Autodesk Inventor part; units mm, degrees
ref_plane "YZ Plane" through (0, 0, 0) normal (1, 0, 0) x (0, 1, 0)
ref_plane "XZ Plane" through (0, 0, 0) normal (0, 1, 0) x (-1, 0, 0)
ref_plane "XY Plane" through (0, 0, 0) normal (0, 0, 1) x (1, 0, 0)
sketch "Boceto2" plane through (0, 0, 0) normal (0, 0, 1) x (1, 0, 0)
  line L0 (-14, 15) -> (0, 15)
  line L1 (3, 8.5) -> (3, 3.5)
  line L2 (0, 0) -> (-14, 0)
  line L3 (-17, 3.5) -> (-17, 8.5)
  line L4 (-14, 8.5) -> (-17, 8.5)
  line L5 (-17, 3.5) -> (-14, 3.5)
  line L6 (0, 8.5) -> (3, 8.5)
  line L7 (0, 3.5) -> (3, 3.5)
  line L8 (-14, 15) -> (-14, 8.5)
  line L9 (-14, 3.5) -> (-14, 0)
  line L10 (0, 15) -> (0, 8.5)
  line L11 (0, 3.5) -> (0, 0)
  point P0 (1.5, 3.5)
  dimension "d4" = 20
  dimension "d5" = 15
  dimension "d9" = 5
  dimension "d10" = 3
  dimension "d11" = 3
  dimension "d12" = 5
  dimension "d15" = 3.5
extrude "Extrusión1" add sketch "Boceto2" along normal blind 3
properties part number "abajo"
Source: CAD feature listing. Evaluate the final solid. Frame: model axes, mm. A direction names the side the tool comes from. Give positions to 0.01 mm unless a question says otherwise; leave off trailing zeros. Order: outer loops, then holes, each group sorted by start corner. A loop starts at its lowest first (then second) coordinate and runs counter-clockwise, first axis right, second up.
(1) Material intervals for line 1 along Y through (x, z) = (-14.75, 0.2); line 2 along X through (y, z) = (1.75, 1.2), sorted ascending.
(2) Section query A-A (z = 1.6). Return the cut outline in (x, y).
(3) Access query for faces 4 (the face through (-15, 8.5, 1)), 5 (the face through (-16, 3.5, 1)), 6 (the face through (0, 12, 1)), 7 (the face through (1, 3.5, 1)), 8 (the face through (-7, 0, 1)). Directions: +Z, -Z, +X, -X, +Y, -Y. A direction counts if a zero-diameter tool reaches every point of the face in a straight line with its end or side. Return the directions, or none.
(4) Contact query for flat-ended pins moving along their axis: P1, Ø1.5, axis at y = 11.5, z = 1, coming from the +X side; P2, Ø1.5, axis at y = 1, z = 1.5, coming from the -X side; P3, Ø1.5, axis at x = 2, z = 1, coming from the +Y side. Output: stop coordinate, or through.
(5) Section query C-C (y = 2). Return the cut outline in (x, z), plus the area to 3 significant figures.
(6) Section query B-B (x = -14.5). Return the cut outline in (y, z).
(7) Pull-direction query (Z, two-part tool) for faces 1 (the face through (-7, 8, 3)), 2 (the face through (-7, 8, 0)), 3 (the face through (1, 8.5, 1)); classes: +Z half, -Z half, draft (parallel to the pull), parting line (faces both ways), or undercut.
Outcome:
1. line 1: y = 3.5 to 8.5
1. line 2: x = -14 to 0
2. outline: (-17, 3.5) - (-14, 3.5) - (-14, 0) - (0, 0) - (0, 3.5) - (3, 3.5) - (3, 8.5) - (0, 8.5) - (0, 15) - (-14, 15) - (-14, 8.5) - (-17, 8.5) - close
3. face 4: +Z, -Z, -X, +Y
3. face 5: +Z, -Z, -X, -Y
3. face 6: +Z, -Z, +X, +Y
3. face 7: +Z, -Z, +X, -Y
3. face 8: +Z, -Z, +X, -X, -Y
4. P1: stops at x = 0
4. P2: stops at x = -14
4. P3: stops at y = 8.5
5. outline: (-14, 0) - (0, 0) - (0, 3) - (-14, 3) - close
5. area: 42.0 mm2
6. outline: (3.5, 0) - (8.5, 0) - (8.5, 3) - (3.5, 3) - close
7. face 1: +Z half
7. face 2: -Z half
7. face 3: draft
